CAD build for the part. Positions are in the model's coordinates, mm. Round coordinates to 2 decimals unless told otherwise and drop trailing zeros. Loops run counter-clockwise (first coordinate to the right, second up) from the corner with the lowest first, then second, coordinate; pieces in that order, holes last.
Autodesk Inventor part; units mm, degrees
ref_plane "YZ Plane" through (0, 0, 0) normal (1, 0, 0) x (0, 1, 0)
ref_plane "XZ Plane" through (0, 0, 0) normal (0, 1, 0) x (-1, 0, 0)
ref_plane "XY Plane" through (0, 0, 0) normal (0, 0, 1) x (1, 0, 0)
sketch "Sketch1" plane through (0, 0, 0) normal (1, 0, 0) x (0, 1, 0)
  line L0 (0, 0) -> (16, 0)
  line L1 (16, 0) -> (16, -100)
  line L2 (16, -100) -> (0, -100)
  line L3 (0, -10) -> (0, -10)
  line L4 (0, -10) -> (0, -25)
  line L5 (0, -25) -> (0, -25)
  line L6 (0, -90) -> (0, -90)
  line L7 (0, -90) -> (0, -75)
  line L8 (0, -75) -> (0, -75)
  line L9 (0, -10) -> (0, 0)
  line L10 (0, -100) -> (0, -90)
  line L11 (0, -75) -> (0, -25)
  dimension "d0" = 16
  dimension "d1" = 100
  dimension "d2" = 0
  dimension "d3" = 15
  dimension "d4" = 10
  dimension "d5" = 15
  dimension "d6" = 10
  dimension "d10" = 0
  dimension "d11" = 0
  dimension "d12" = 0
extrude "Extrusion1" add sketch "Sketch1" along normal blind 2
sketch "Sketch5" plane through (2, 0, 0) normal (1, 0, 0) x (0, 0, -1)
  line L0 (0, 0) -> (100, 0)
  circle A0 centre (63.5, -19) radius 2.5
  line L1 (56.5, 0) -> (72.5, 0)
  line L2 (72.5, 0) -> (72.5, -25)
  line L3 (72.5, -25) -> (56.5, -25)
  line L4 (56.5, -25) -> (56.5, 0)
  circle A1 centre (66.2831, 1.8148) radius 2.5
  circle A2 centre (56, 8) radius 6 construction
  circle A3 centre (63.5, -19) radius 15 construction
  circle A4 centre (66.2831, 1.8148) radius 6 construction
  dimension "d44" = 16
  dimension "d45" = 25
  dimension "d46" = 9
  dimension "d52" = 5
  dimension "d56" = 12
  dimension "d57" = 30
  dimension "d58" = 12
extrude "Extrusion6" add sketch "Sketch5" against normal blind 2 contours L0 A1 L2 L3 L4 | L0 A1 picked at (65.8534, -0.1091)
sketch "Sketch7" plane through (2, 0, 0) normal (1, 0, 0) x (0, 0, -1)
  circle A0 centre (44, 8) radius 2.5
  circle A1 centre (56, 8) radius 2.5
  circle A2 centre (66.2831, 1.8148) radius 2.5
  circle A3 centre (63.5, -19) radius 2.5
  circle A4 centre (44, 8) radius 2.5
  circle A5 centre (56, 8) radius 2.5
  circle A6 centre (66.2831, 1.8148) radius 2.5
  circle A7 centre (63.5, -19) radius 2.5
  circle A8 centre (63.5, -19) radius 2.5
  point P0 (0, 0)
  dimension "d59" = 5
  dimension "d60" = 5
  dimension "d61" = 5
  dimension "d62" = 5
extrude "Extrusion8" cut sketch "Sketch7" against normal blind 10 contours A0 | A1 | A2
sketch "Sketch8" plane through (2, 0, 0) normal (1, 0, 0) x (0, 0, -1)
  circle A0 centre (44, 8) radius 2.5
  line L0 (0, 0) -> (56.5, 0)
  line L1 (0, 16) -> (0, 0)
  line L2 (100, 16) -> (0, 16)
  line L3 (56.5, 0) -> (0, 0)
  line L4 (34, 0) -> (0, 0)
  line L5 (0, 0) -> (0, 16)
  line L6 (0, 16) -> (34, 16)
  line L7 (34, 16) -> (34, 0)
  dimension "d65" = 10
extrude "Extrusion9" cut sketch "Sketch8" against normal blind 10 contours L1 L2 L7 L0
sketch "Sketch9" plane through (2, 0, 0) normal (1, 0, 0) x (0, 0, -1)
  circle A0 centre (56, 8) radius 2.5
  circle A1 centre (66.2831, 1.8148) radius 2.5
  circle A2 centre (65, 7.8652) radius 2.5
  circle A3 centre (86, 7.8652) radius 2.5
  circle A4 centre (44, 8) radius 2.5
  point P0 (0, 0)
  dimension "d68" = 5
  dimension "d71" = 5
  dimension "d72" = 21
  dimension "d76" = 21
  dimension "d77" = 6.0505
  dimension "d78" = 6.0505
extrude "Extrusion10" cut sketch "Sketch9" against normal blind 10 contours A2 | A3
sketch "Sketch10" plane through (0, 0, 0) normal (-1, 0, 0) x (0, 0, 1)
  line L0 (-123.9658, 20.3206) -> (-103.1897, 17.2622)
  line L1 (-124.0249, -0.6793) -> (-123.9658, 20.3206)
  line L2 (-102.025, -0.7412) -> (-124.0249, -0.6793)
  line L3 (-102.025, -0.7412) -> (-101.9743, 17.2588)
  line L4 (-103.1897, 17.2622) -> (-101.9743, 17.2588)
  circle A0 centre (-65, 7.8652) radius 2.5
  circle A1 centre (-86, 7.8652) radius 2.5
  line L5 (-34, 0) -> (-34, 16)
  line L6 (-34, 16) -> (-100, 16)
  line L7 (-100, 16) -> (-100, 0)
  line L8 (-100, 0) -> (-72.5, 0)
  line L9 (-72.5, 0) -> (-72.5, -25)
  line L10 (-72.5, -25) -> (-56.5, -25)
  line L11 (-56.5, -25) -> (-56.5, 0)
  line L12 (-56.5, 0) -> (-34, 0)
  circle A2 centre (-63.5, -19) radius 2.5
  circle A3 centre (-66.2831, 1.8148) radius 2.5
  circle A4 centre (-44, 8) radius 2.5
  circle A5 centre (-56, 8) radius 2.5
  line L13 (-100, 16) -> (-123, 16)
  line L14 (-123, 16) -> (-123, 0)
  line L15 (-123, 0) -> (-100, 0)
  line L16 (-100, 0) -> (-100, 16)
  point P0 (0, 0)
  dimension "d79" = 23
extrude "Extrusion11" add sketch "Sketch10" against normal blind 2 contours L13 L7 L15 L3 | L3 L15 L14 L13
sketch "Sketch11" plane through (2, 0, 0) normal (1, 0, 0) x (0, 0, -1)
  circle A0 centre (110, 7.8652) radius 2.5
  circle A1 centre (110, 7.8652) radius 2.5
  point P0 (0, 0)
  dimension "d82" = 5
extrude "Extrusion12" cut sketch "Sketch11" against normal blind 10
equation "\"d78\" = d77"
properties part number "Mounting_wall_3"
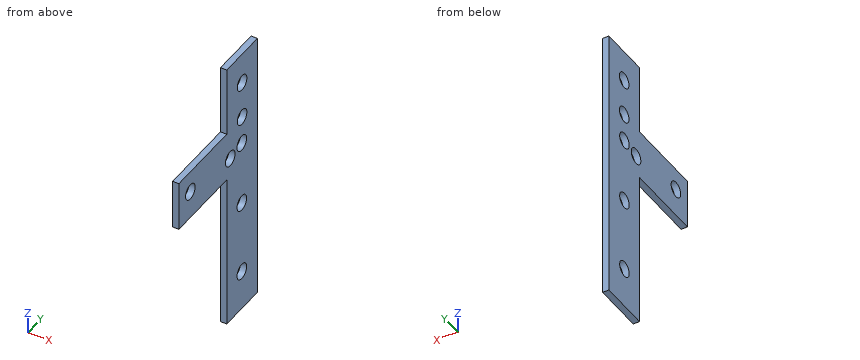
Item 1: Wall check: L1, parallel to Y at x = 0.6, z = -110; L2, parallel to Z at x = 1.6, y = 9.5; L3, parallel to Z at x = 0.5, y = -1. Give the ranges that are in metal, low to high.
Verdict:
L1: y = 0 to 5.37, 10.37 to 16
L2: z = -123 to -111.89, -108.11 to -87.89, -84.11 to -66.89, -63.11 to -58, -54 to -46, -42 to -34
L3: z = -72.5 to -56.5
Item 2: Cut at B-B (z = -110). List the corners of the cut face in (x, y).
Verdict:
outline: (0, 0) - (2, 0) - (2, 5.37) - (0, 5.37) - close; (0, 10.37) - (2, 10.37) - (2, 16) - (0, 16) - close
Item 3: Cut at A-A (y = -19). List the corners of the cut face in (x, z).
Verdict:
outline: (0, -72.5) - (2, -72.5) - (2, -66) - (0, -66) - close; (0, -61) - (2, -61) - (2, -56.5) - (0, -56.5) - close
Item 4: Cut at C-C (x = 0.75). List the corners of the cut face in (y, z).
Verdict:
outline: (-25, -72.5) - (0, -72.5) - (0, -123) - (16, -123) - (16, -34) - (0, -34) - (0, -56.5) - (-25, -56.5) - close; hole circle Ø5 at (-19, -63.5); hole circle Ø5 at (1.81, -66.28); hole circle Ø5 at (7.87, -110); hole circle Ø5 at (7.87, -86); hole circle Ø5 at (7.87, -65); hole circle Ø5 at (8, -56); hole circle Ø5 at (8, -44)
Item 5: Flat gauge pins, fed straight in: P1, Ø4.5, axis at y = 8, z = -56, coming from the -X side; P2, Ø0.6, axis at x = 1.5, y = -13.5, coming from the +Z side; P3, Ø1, axis at x = 1, y = -9, coming from the -Z side. Where does each tip first touch, or does it go through?
Verdict:
P1: passes through
P2: stops at z = -56.5
P3: stops at z = -72.5
Item 6: Cut at D-D (z = -98.5). List the corners of the cut face in (x, y).
Verdict:
outline: (0, 0) - (2, 0) - (2, 16) - (0, 16) - close
